Geometry: final body of the model. Coordinates: model frame, mm. A direction names the side the tool comes from. Give positions to 0.01 mm unless a question says otherwise; leave off trailing zeros. Write each loop counter-clockwise with the first axis right and the second up, starting at its lowest first coordinate (ties: lowest second). Pieces come first, ordered by that corner, then holes. Notation, with made-up numbers: (29.5, -32) - (86.5, -32) arc R37 ccw to (86.5, 4) - close; hole circle Ø9 at (-35.5, -7). An arc over 180 degrees is marked (long way). Return JSON: item names as keys, results as strings.
Autodesk Inventor part; units mm, degrees
ref_plane "YZ Plane" through (0, 0, 0) normal (1, 0, 0) x (0, 1, 0)
ref_plane "XZ Plane" through (0, 0, 0) normal (0, 1, 0) x (-1, 0, 0)
ref_plane "XY Plane" through (0, 0, 0) normal (0, 0, 1) x (1, 0, 0)
sketch "Náčrt1" plane through (0, 0, 0) normal (0, 0, 1) x (1, 0, 0)
  line L0 (1.3202, 0) -> (0, 0)
  line L1 (0, 0) -> (0, 10)
  line L2 (0, 10) -> (0.5, 10)
  line L3 (0.5, 10) -> (0.5, 0.5)
  line L4 (0.5, 0.5) -> (10, 0.5)
  line L5 (10, 0.5) -> (10, 0)
  line L6 (10, 0) -> (1.3202, 0)
  point P0 (10, 0.25)
  point P1 (0.25, 10)
  dimension "d0" = 0.5
  dimension "d1" = 0.5
  dimension "d2" = 10
  dimension "d3" = 10
extrude "Vysunutí1" add sketch "Náčrt1" along normal blind 10
sketch "Náčrt2" plane through (0.5, 0.5, 0) normal (0, 1, 0) x (1, 0, 0)
  line L0 (9.5, 0) -> (0, 0)
  line L1 (9.5, 0) -> (9.5, -10)
  line L2 (2.2639, -3) -> (6.7361, -3)
  line L3 (2.2639, -7) -> (6.7361, -7)
  arc A0 (2.2639, -3) -> (2.2639, -7) centre (4.5, -5) ccw
  arc A1 (6.7361, -7) -> (6.7361, -3) centre (4.5, -5) ccw
  point P0 (-0.5, 0)
  point P1 (4.8669, -7)
  dimension "d7" = 5
  dimension "d8" = 5
  dimension "d9" = 2
  dimension "d10" = 4
extrude "Vysunutí2" cut sketch "Náčrt2" against normal through all
pattern_linear "Obdélníkové pole1" count 10 spacing 10 along (0, 0, 1) of "Vysunutí2"
sketch "Náčrt4" plane through (0.5, 0.5, 0) normal (1, 0, 0) x (0, 0, -1)
  line L0 (0, 0) -> (0, 9.5)
  line L1 (0, 9.5) -> (-10, 9.5)
  line L2 (-10, 0) -> (-10, 9.5)
  circle A0 centre (-5, 4.5) radius 2
  point P0 (0, -0.5)
  point P1 (-5, 9.5)
  point P2 (0, 4.5)
  point P3 (-10, 4.5)
  point P4 (-95, 9.5)
  dimension "d30" = 4
extrude "Vysunutí4" cut sketch "Náčrt4" against normal blind 10
sketch "Náčrt5" plane through (0.5, 0.5, 10) normal (1, 0, 0) x (0, 0, -1)
  circle A0 centre (5, 4.5) radius 2
  line L0 (10, 9.5) -> (0, 9.5)
  line L1 (0, 0) -> (0, 9.5)
  point P0 (10, -0.5)
  point P1 (95, 9.5)
  point P2 (5, 9.5)
  point P3 (0, 4.5)
  dimension "d33" = 4
  dimension "d34" = 5
  dimension "d35" = 5
extrude "Vysunutí5" cut sketch "Náčrt5" against normal blind 10
pattern_linear "Obdélníkové pole3" count 10 spacing 10 along (0, 0, -1) of "Vysunutí5"
sketch "Náčrt6" plane through (0.5, 0.5, 0) normal (0, 1, 0) x (1, 0, 0)
  circle A0 centre (4.5, -5) radius 5
  line L0 (9.5, 0) -> (9.5, -10)
  line L1 (9.5, -10) -> (0, -10)
  line L2 (-0.5, 0) -> (9.5, 0)
  line L3 (9.5, 0) -> (0, 0)
  line L4 (4.5, 0) -> (9.5, 0)
  line L5 (9.5, 0) -> (9.5, -10)
  point P0 (4.5, 0)
  point P1 (9.5, -5)
  point P2 (4.5, -10)
  dimension "d44" = 10
  dimension "d45" = 5
  dimension "d46" = 5
extrude "Vysunutí6" cut sketch "Náčrt6" against normal blind 10 contours L0 L1 A0 | A0 L2 L0
sketch "Náčrt7" plane through (0.5, 0.5, 0) normal (1, 0, 0) x (0, 0, -1)
  circle A0 centre (-5, 4.5) radius 5
  line L0 (0, 0) -> (0, 9.5)
  line L1 (-10, 0) -> (-10, 9.5)
  line L2 (0, 9.5) -> (-10, 9.5)
  point P0 (0, -0.5)
  point P1 (-5, 9.5)
  point P2 (0, 4.5)
  point P3 (-10, 4.5)
  dimension "d49" = 10
  dimension "d50" = 5
  dimension "d51" = 5
  dimension "d52" = 5
extrude "Vysunutí7" cut sketch "Náčrt7" against normal blind 10 contours A0 L2 L0 | A0 L1 L2
properties part number "1001"
Q1. Section query D-D, the plane z = 8.75. Return the cut outline in (x, y), plus the area to 3 significant figures.
Answer key:
{"outline": "(0, 0) - (8.31, 0) - (8.31, 0.5) - (0.5, 0.5) - (0.5, 8.31) - (0, 8.31) - close", "area": "8.06 mm^2"}
Q2. Set-up query: faces 4 (the flat face through (0.5, 3, 6)), 5 (the cylindrical face through (0.3, 10, 4.9)). Return all of +Z, -Z, +X, -X, +Y, -Y with unobstructed straight access to the full face (end or side cutting, diameter ignored); none if empty.
Answer key:
{"face 4": "+Z, -Z, +X, +Y", "face 5": "+X, -X, +Y"}
Q3. Mould query, pull axis Z, two halves, no side actions, for faces 1 (the cylindrical face through (0.254, 5.088, 6.998)), 2 (the cylindrical face through (10, 0.3, 5.1)), 3 (the flat face through (5.2, 0.5, 7.2)). Classes: pulls with the +Z half, pulls with the -Z half, needs draft (parallel to the pull), parting line crosses it, or undercut.
Answer key:
{"face 1": "undercut", "face 2": "parting line crosses it", "face 3": "needs draft"}
Q4. Pin query (flat end, axial travel): P1, Ø5, axis at x = 4, z = 9, coming from the +Y side; P2, Ø6, axis at y = 8, z = 5, coming from the +X side. Return the tip coordinate at first contact, or that it passes through.
Answer key:
{"P1": "stops at y = 0.5", "P2": "stops at x = 0.5"}
Q5. Section query A-A, the plane z = 5. Return the cut outline in (x, y), plus the area to 3 significant figures.
Answer key:
{"outline": "(0, 0) - (2, 0) - (2, 0.5) - (0.5, 0.5) - (0.5, 3) - (0, 3) - close; (0, 7) - (0.5, 7) - (0.5, 10) - (0, 10) - close; (8, 0) - (10, 0) - (10, 0.5) - (8, 0.5) - close", "area": "4.75 mm^2"}
Q6. Section query C-C, the plane y = 5.75. Return the cut outline in (x, z), plus the area to 3 significant figures.
Answer key:
{"outline": "(0, 0.06) - (0.5, 0.06) - (0.5, 3.15) - (0, 3.15) - close; (0, 6.85) - (0.5, 6.85) - (0.5, 9.94) - (0, 9.94) - close", "area": "3.09 mm^2"}
Q7. Material intervals for probe 1 along Y at (x, z) = (0.3, 5); probe 2 along X at (y, z) = (7.25, 8.5), sorted ascending. Write a range as [from, to].
Answer key:
{"probe 1": "y = [0, 3], [7, 10]", "probe 2": "x = [0, 0.5]"}
Q8. Section query B-B, the plane x = 3.75. Return the cut outline in (y, z), plus the area to 3 significant figures.
Answer key:
{"outline": "(0, 0) - (0.5, 0) - (0.5, 3) - (0, 3) - close; (0, 7) - (0.5, 7) - (0.5, 10) - (0, 10) - close", "area": "3.00 mm^2"}
